Job drawing, mm, ordinate dimensions from the low corner. One solid piece. A direction names the side the tool comes from. Round coordinates to 2 decimals unless told otherwise and drop trailing zeros. Loops run counter-clockwise (first coordinate to the right, second up) from the corner with the lowest first, then second, coordinate; pieces in that order, holes last. Notation, with made-up numbers: M -14.75,89 L -1.75,89 A19 ccw -1.75,104 Z; hole C -8,37.5 d11. An arc over 180 degrees is marked long. Put each result on its own line as item: value. Start each with the question number.
1) Slice it at C-C on z = 5.5. Give the cut face in (x, y).
2) Probe line 1 along Z through (x, y) = (1.5, 12.75); line 2 along Y through (x, z) = (10, 9.75) (3 decimals); line 3 along Y through (x, z) = (10, 3.5). List the from-to ranges inside material, lowest first.
3) Drop flat-ended pins along their axis: pin 1 Ø1.5 at (y, z) = (15, 7) entering from -X; pin 2 Ø5 at (x, y) = (7, 9) entering from +Z; pin 3 Ø1 at (y, z) = (16, 7.5) entering from -X. Give the stop position or say it passes through.
4) Slice it at A-A on x = 10. Give the cut face in (y, z) (3 decimals), then the cut area to 4 significant figures.
5) Pull direction Z, two halves, no side cores. Call the marked faces 1, 2, 3 and 4: +Z half, -Z half, draft (parallel to the pull), parting line (faces both ways), or undercut.
6) Slice it at D-D on z = 3. Give the cut face in (x, y).
7) Which spindle directions (+Z, -Z, +X, -X, +Y, -Y) get a long thin tool onto all of the face, cutting with end or side? Do the marked faces 5 and 6. Say none if no direction does.
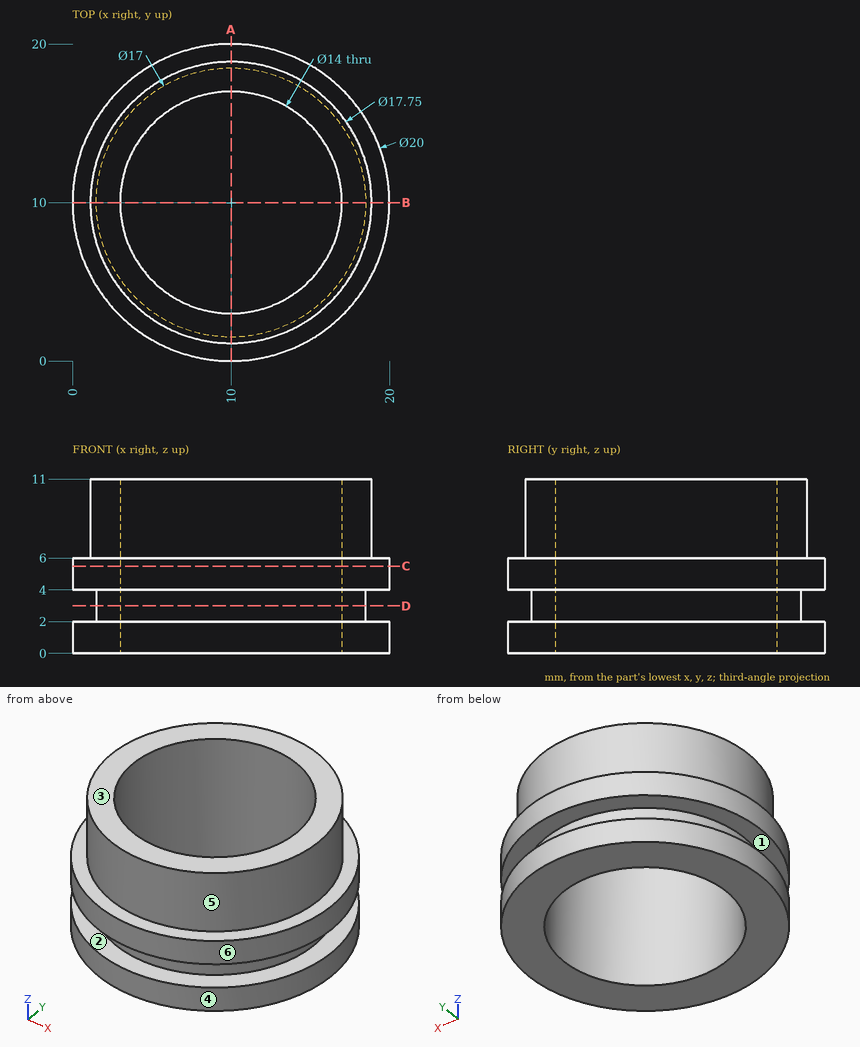
Recorded:
1. outline: C 10,10 d20; hole C 10,10 d14
2. line 1: z = 0 to 2, 4 to 6
2. line 2: y = 1.125 to 3, 17 to 18.875
2. line 3: y = 1.5 to 3, 17 to 18.5
3. pin 1: stops at x = 2.21
3. pin 2: passes through
3. pin 3: stops at x = 3.03
4. outline: M 0,0 L 3,0 L 3,11 L 1.125,11 L 1.125,6 L 0,6 L 0,4 L 1.5,4 L 1.5,2 L 0,2 Z; M 17,0 L 20,0 L 20,2 L 18.5,2 L 18.5,4 L 20,4 L 20,6 L 18.875,6 L 18.875,11 L 17,11 Z
4. area: 48.75 mm2
5. face 1: undercut
5. face 2: undercut
5. face 3: +Z half
5. face 4: draft
6. outline: C 10,10 d17; hole C 10,10 d14
7. face 5: +Z
7. face 6: +Z, -Z
